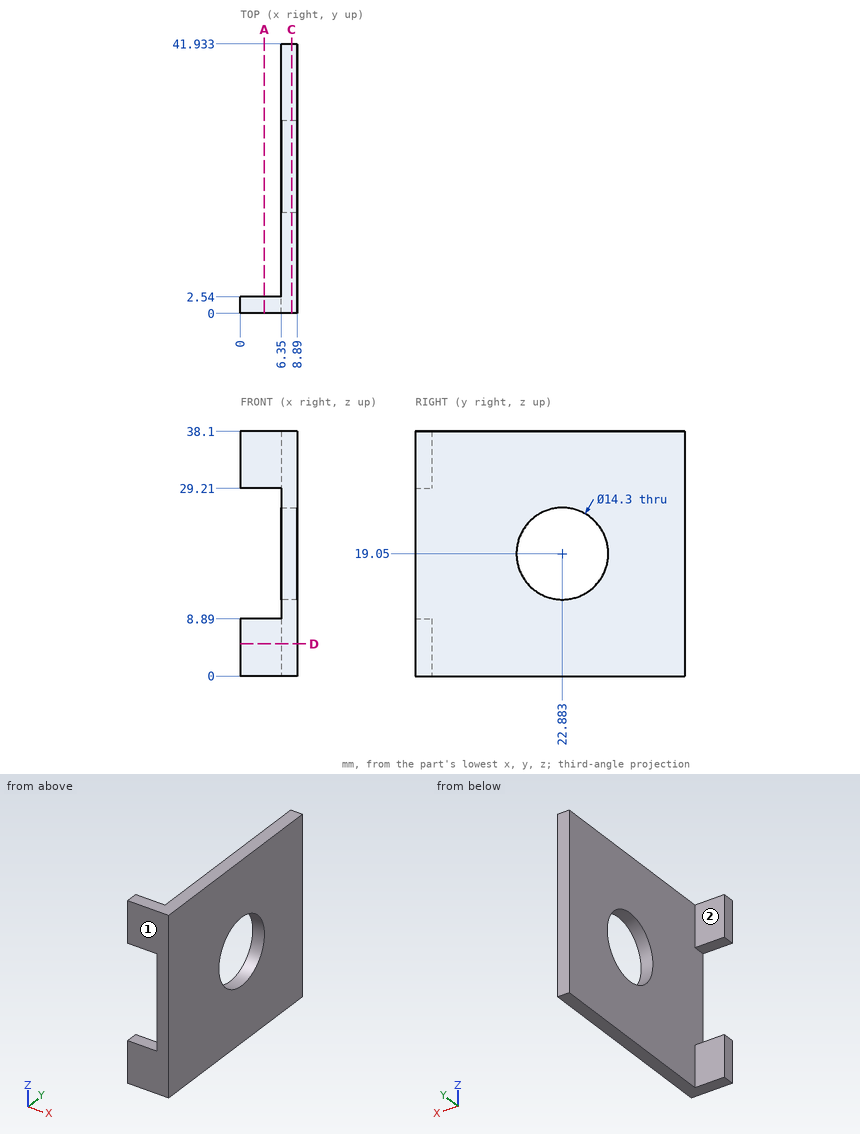
Geometry: see drawing. Coordinates: mm, zero at the bounding-box minimum. A direction names the side the tool comes from. Round coordinates to 2 decimals unless told otherwise and drop trailing zeros. Write each loop counter-clockwise with the first axis right and the second up, starting at its lowest first coordinate (ties: lowest second). Pieces come first, ordered by that corner, then holes. Notation, with made-up numbers: M 7.5,42.25 L 17.5,42.25 A31 ccw 17.5,77.25 Z; hole C 78.5,-34.75 d4. An arc over 180 degrees is marked long. Answer as a JSON object with one key per item and string values. Group by question number.
(1) Section query A-A on x = 3.75. Output: boundary loops of the cut face in (y, z).
(2) Reachability of the marked faces 1 and 2 from +Z, -Z, +X, -X, +Y, -Y: full face, straight path, thin tool, end or side. Return the list, or none.
(3) Section query C-C on x = 8. Output: boundary loops of the cut face in (y, z), then the cut area to 3 significant figures.
(4) First-contact query: pin 1 (1.9 mm diameter, centred on x = 4, z = 6.5, fed in from +Y); pin 2 (11.5 mm diameter, centred on y = 24, z = 27.5, fed in from -X). Flat tips, straight axial feed; report the tip coordinate or a pass-through.
(5) Ray query, line 1 (Y direction, x = 7.6, z = 19.05); line 2 (X direction, y = 19, z = 26); line 3 (Y direction, x = 6, z = 7.5). Return the intervals inside material, ascending. Write a range as [from, to].
(6) Section query D-D on z = 5. Output: boundary loops of the cut face in (x, y), then the cut area to 3 significant figures.
Computed values:
{
 "1": {"outline": "M 0,0 L 2.54,0 L 2.54,8.89 L 0,8.89 Z; M 0,29.21 L 2.54,29.21 L 2.54,38.1 L 0,38.1 Z"},
 "2": {"face 1": "+Z, -Z, +X, -X, -Y", "face 2": "+Z, -Z, -X, +Y"},
 "3": {"outline": "M 0,0 L 41.93,0 L 41.93,38.1 L 0,38.1 Z; hole C 22.88,19.05 d14.3", "area": "1,440 mm^2"},
 "4": {"pin 1": "y = 2.54", "pin 2": "x = 6.35"},
 "5": {"line 1": "[0, 15.73], [30.03, 41.93]", "line 2": "[6.35, 8.89]", "line 3": "[0, 2.54]"},
 "6": {"outline": "M 0,0 L 8.89,0 L 8.89,41.93 L 6.35,41.93 L 6.35,2.54 L 0,2.54 Z", "area": "123 mm^2"}
}
